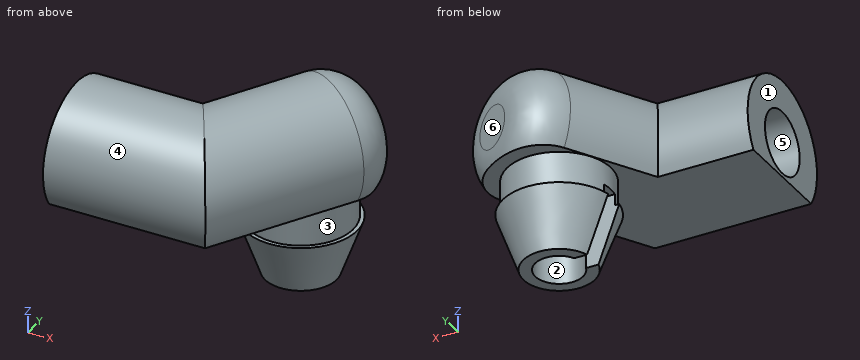
from build123d import *

# Parameters (mm, degrees)
SKETCH3_R           = 2.25
FILLET2_R           = 1.5
SKETCH4_R           = 1.125
SKETCH6_W           = 9.297020352
SKETCH6_H           = 8.256436423
CUT_EXTRUDE1_DEPTH  = 3
SKETCH7_R           = 1.85
BOSS_EXTRUDE2_DEPTH = 1.2
SKETCH8_R           = 2
BOSS_EXTRUDE3_DEPTH = 2
BOSS_EXTRUDE3_TAPER = 20
SKETCH9_R           = 0.85
CUT_EXTRUDE2_DEPTH  = 2.4
SKETCH10_W          = 1.535398486
SKETCH10_H          = 0.7
CUT_EXTRUDE3_DEPTH  = 2.4


with BuildPart() as part:
    # Sweep1: sweep along a path in Sketch2
    with BuildLine(Plane.XY) as sweep1_path:
        Line((-4.5, 0), (0, 0))
        Line((0, 0), (3, 5.196152423))
    # Sketch3 → Sweep1 (sweep)
    with BuildSketch(Plane(origin=(-4.5, 0, 0), x_dir=(0, 0, -1), z_dir=(1, 0, 0))):
        Circle(SKETCH3_R)
    sweep(path=sweep1_path.line, transition=Transition.RIGHT)

    # Fillet2
    fillet2_edges = [part.edges().sort_by_distance(p)[0] for p in [
        (3, 5.196152423, 2.25),
    ]]
    fillet(fillet2_edges, radius=FILLET2_R)

    # Cut-Sweep1: sweep along a path in Sketch5
    with BuildLine(Plane.XY) as cut_sweep1_path:
        Line((-4.5, 0), (1.2, 0))
    # Sketch4 → Cut-Sweep1 (sweep, cut)
    with BuildSketch(Plane.ZY.offset(4.5)):
        Circle(SKETCH4_R)
    sweep(path=cut_sweep1_path.line, mode=Mode.SUBTRACT)

    # Sketch6 → Cut-Extrude1 (cut)
    with BuildSketch(Plane.XY.offset(-1.25)):
        with Locations((-0.019421036, 1.725207659)):
            Rectangle(SKETCH6_W, SKETCH6_H)
    extrude(amount=-CUT_EXTRUDE1_DEPTH, mode=Mode.SUBTRACT)

    # Sketch7 → Boss-Extrude2 (add)
    with BuildSketch(Plane(origin=(0, 0, -1.25), x_dir=(-1, 0, 0), z_dir=(0, 0, -1))):
        with Locations(Location((-1.777414459, 3.078572149, 0), (0, 0, 180))):
            Circle(SKETCH7_R)
    extrude(amount=BOSS_EXTRUDE2_DEPTH)

    # Sketch8 → Boss-Extrude3 (add)
    with BuildSketch(Plane(origin=(0, 0, -2.45), x_dir=(-1, 0, 0), z_dir=(0, 0, -1))):
        with Locations((-1.777414459, 3.078572149)):
            Circle(SKETCH8_R)
    extrude(amount=BOSS_EXTRUDE3_DEPTH, taper=BOSS_EXTRUDE3_TAPER)

    # Sketch9 → Cut-Extrude2 (cut)
    with BuildSketch(Plane(origin=(0, 0, -4.45), x_dir=(-1, 0, 0), z_dir=(0, 0, -1))):
        with Locations((-1.777414459, 3.078572149)):
            Circle(SKETCH9_R)
    extrude(amount=-CUT_EXTRUDE2_DEPTH, mode=Mode.SUBTRACT)

    # Sketch10 → Cut-Extrude3 (cut)
    with BuildSketch(Plane(origin=(0, 0, -4.45), x_dir=(-1, 0, 0), z_dir=(0, 0, -1))):
        with Locations((-0.333609148, 3.11663504)):
            Rectangle(SKETCH10_W, SKETCH10_H)
    extrude(amount=-CUT_EXTRUDE3_DEPTH, mode=Mode.SUBTRACT)


solid = part.part
Read the model definition and answer for the solid it produces. Units are mm, in the model's axes. Face numbers are marked on the shaded views. A direction names the side the tool comes from. Coordinates: 2 decimals unless noted, no trailing zeros. Order: outer loops, then holes, each group sorted by start corner. A loop starts at its lowest first (then second) coordinate and runs counter-clockwise, first axis right, second up. Notation, with made-up numbers: M -24.75,89 L -5.75,89 A25 ccw -5.75,125 Z; hole C 87,-35.75 d6. An arc over 180 degrees is marked long. Put each result on its own line as item: value. Start each with the question number.
Item 1: Given pin 1 Ø3 at (x, y) = (1, -1) entering from -Z; pin 2 Ø1.2 at (x, y) = (1.5, 4) entering from +Z; pin 3 Ø3 at (x, z) = (0.5, -1) entering from +Y; pin 4 Ø1.3 at (x, z) = (0.5, -3) entering from +Y, each flat-ended and moving along its own axis, determine where each tip first touches the part or whether it passes through.
Item 2: Consider probe 1 along Y at (x, z) = (1.75, -2.25); probe 2 along Y at (x, z) = (-1.5, -0.5); probe 3 along X at (y, z) = (2.5, -3.5). Determine where each line is inside the solid, lowest interval first. Write a range as [from, to].
Item 3: Section A-A, the plane z = -2.75 is taken. Determine the outline of the cut face in (x, y).
Item 4: For the marked faces 1, 2 and 3, determine the directions among +Z, -Z, +X, -X, +Y, -Y from which every point of the face is accessible in a straight line to the end or side of a thin tool.
Item 5: The mould has two halves that part along Z. Classify the marked faces 4, 5 and 6: +Z half, -Z half, draft (parallel to the pull), parting line (faces both ways), or undercut.
Computed:
1. pin 1: stops at z = -1.25
1. pin 2: stops at z = 2.25
1. pin 3: stops at y = 5.77
1. pin 4: stops at y = 4.87
2. probe 1: y = [1.23, 2.23], [3.93, 4.93]
2. probe 2: y = [-2.19, -1.01], [1.01, 2.19]
2. probe 3: x = [0.27, 1.15], [2.4, 3.29]
3. outline: M -0.09,2.77 A1.89 ccw long -0.07,3.47 L 1.02,3.47 A0.85 cw long 0.99,2.77 Z
4. face 1: +Z, -Z, -X, +Y, -Y
4. face 2: -Z
4. face 3: none
5. face 4: parting line
5. face 5: undercut
5. face 6: draft
